from build123d import *

# Parameters (mm, degrees)
BOSS_EXTRUDE2_DEPTH = 7
SKETCH4_W           = 24
SKETCH4_H           = 4
CUT_EXTRUDE1_DEPTH  = 13


with BuildPart() as part:
    # Sketch3 → Boss-Extrude2 (new body)
    with BuildSketch(Plane(origin=(0, 0, 0), x_dir=(1, 0, 0), z_dir=(0, 1, 0))):
        Polygon((12, 11.5), (-12, 11.5), (-12, 1.5), (2, 1.5), (2, -11.5), (12, -11.5), align=None)
    extrude(amount=-BOSS_EXTRUDE2_DEPTH)

    # Sketch4 → Cut-Extrude1 (cut)
    with BuildSketch(Plane.XY.offset(11.5)):
        with Locations((0, -3.5)):
            Rectangle(SKETCH4_W, SKETCH4_H)
    extrude(amount=-CUT_EXTRUDE1_DEPTH, mode=Mode.SUBTRACT)


solid = part.part
Build history of the part. All positions in model axes, mm. A direction names the side the tool comes from. Round coordinates to 2 decimals unless told otherwise and drop trailing zeros. Loops run counter-clockwise (first coordinate to the right, second up) from the corner with the lowest first, then second, coordinate; pieces in that order, holes last. Notation, with made-up numbers: (29, 5.5) -> (74, 5.5) arc R15 cw to (74, 18.5) -> close; hole circle Ø10 at (54, -11). An arc over 180 degrees is marked (long way). Answer in a Markdown table with one row per item.
Item 1: Mould opens along Y. For faces 1 (the flat face through (2, -7, -3)), 2 (the flat face through (7, -1, 11.5)), 3 (the flat face through (7, -5.5, 5)) say: +Y half, -Y half, draft (parallel to the pull), parting line (faces both ways), or undercut.
Answers below:
| item | result |
|---|---|
| face 1 | -Y half |
| face 2 | draft |
| face 3 | undercut |
Item 2: Drill centre lines: L1, parallel to Y at x = 8, z = -0.75; L2, parallel to Z at x = 7.5, y = -4; L3, parallel to X at y = -6.5, z = 5.25. Where is each one in solid material? Low to high. Write a range as [from, to].
Answers below:
| item | result |
|---|---|
| L1 | y = [-7, -5.5], [-1.5, 0] |
| L2 | z = [-11.5, -1.5] |
| L3 | x = [2, 12] |
Item 3: Saw through at C-C (y = -4.5). Write the cut outline in (x, z).
Answers below:
| item | result |
|---|---|
| outline | (-12, -11.5) -> (12, -11.5) -> (12, -1.5) -> (-12, -1.5) -> close |
Item 4: Saw through at B-B (x = 5.5). Write the cut outline in (y, z).
Answers below:
| item | result |
|---|---|
| outline | (-7, -11.5) -> (0, -11.5) -> (0, 11.5) -> (-1.5, 11.5) -> (-1.5, -1.5) -> (-5.5, -1.5) -> (-5.5, 11.5) -> (-7, 11.5) -> close |
Item 5: Which spindle directions (+Z, -Z, +X, -X, +Y, -Y) get a long thin tool onto all of the face, cutting with end or side? Do faces 4 (the flat face through (2, -6, 5)), 5 (the flat face through (12, -3, -2)), 6 (the flat face through (7, -1.5, 5)). Say none if no direction does.
Answers below:
| item | result |
|---|---|
| face 4 | +Z, -X, +Y, -Y |
| face 5 | +Z, -Z, +X, +Y, -Y |
| face 6 | +Z, +X, -X |
Item 6: Saw through at D-D (x = -2.75). Write the cut outline in (y, z).
Answers below:
| item | result |
|---|---|
| outline | (-7, -11.5) -> (0, -11.5) -> (0, -1.5) -> (-7, -1.5) -> close |
Item 7: Pin check, flat tips, straight feed: pin 1 (12 mm diameter, centred on x = 3, z = -8, fed in from +Y); pin 2 (1.6 mm diameter, centred on y = -6.5, z = 2, fed in from -X). Stop position of each tip, or through.
Answers below:
| item | result |
|---|---|
| pin 1 | stops at y = 0 |
| pin 2 | stops at x = 2 |
Item 8: Saw through at A-A (z = 7.75). Write the cut outline in (x, y).
Answers below:
| item | result |
|---|---|
| outline | (2, -7) -> (12, -7) -> (12, -5.5) -> (2, -5.5) -> close; (2, -1.5) -> (12, -1.5) -> (12, 0) -> (2, 0) -> close |
